Read the model definition and answer for the solid it produces. Units are mm, in the model's axes. Face numbers are marked on the shaded views. A direction names the side the tool comes from. Give positions to 0.01 mm unless a question says otherwise; leave off trailing zeros. Write each loop counter-clockwise with the first axis right and the second up, starting at its lowest first coordinate (ties: lowest second). Pieces come first, ordered by that corner, then holes. Notation, with made-up numbers: M -19,2 L 15,2 A19 ccw 15,12 Z; hole C 68,33.25 d5. An arc over 180 degrees is marked long. Answer as CSV lines item,"result". Start each with the question number.
Autodesk Inventor part; units mm, degrees
ref_plane "YZ Plane" through (0, 0, 0) normal (1, 0, 0) x (0, 1, 0)
ref_plane "XZ Plane" through (0, 0, 0) normal (0, 1, 0) x (-1, 0, 0)
ref_plane "XY Plane" through (0, 0, 0) normal (0, 0, 1) x (1, 0, 0)
sketch "Sketch1" plane through (0, 0, 0) normal (0, 0, 1) x (1, 0, 0)
  line L0 (0, 0) -> (0, 38.4841) construction
  line L1 (2.8, 25) -> (3.8, 24)
  line L2 (3.8, 24) -> (3.8, 0)
  line L3 (2.8, 25) -> (1.4, 25)
  line L4 (1.4, 25) -> (1.4, 0)
  line L5 (1.4, 0) -> (3.8, 0)
  dimension "d1" = 1.4
  dimension "d8" = 1
  dimension "d20" = 3.8
revolve "Revolution1" add sketch "Sketch1" angle 360 about axis through (0, 0, 0) along (0, 1, 0)
chamfer "Chamfer1" distance 0.5 angle 45 2 edges at (-1.4, 25, 0) (-1.4, 0, 0)
sketch "Sketch6" plane through (0, 0, 0) normal (0, -1, 0) x (1, 0, 0)
  line L0 (0, 0) -> (0, -8) construction
  circle A0 centre (0, 8) radius 3
  circle A1 centre (0, -8) radius 3
  circle A2 centre (0, 0) radius 6
  line L1 (0, 0) -> (0, 8) construction
  circle A3 centre (0, 8) radius 1.35
  circle A4 centre (0, -8) radius 1.35
  circle A5 centre (0, 0) radius 1.9
  point P0 (1.9111, -5.6875)
  point P1 (1.9111, 5.6875)
  point P2 (-1.9111, 5.6875)
  point P3 (-1.9111, -5.6875)
  dimension "d24" = 6
  dimension "d26" = 8
  dimension "d27" = 12
  dimension "d28" = 2.7
extrude "Extrusion3" add sketch "Sketch6" against normal blind 8
fillet "Fillet1" radius 4 4 edges at (1.9111, 4, 5.6875) (-1.9111, 4, 5.6875) (1.9111, 4, -5.6875) (-1.9111, 4, -5.6875)
fillet "Fillet2" radius 0.5 4 edges at (0, 8, -11) (6, 8, 0) (-6, 8, 0) (0, 8, 11)
properties part number "caster-bng"
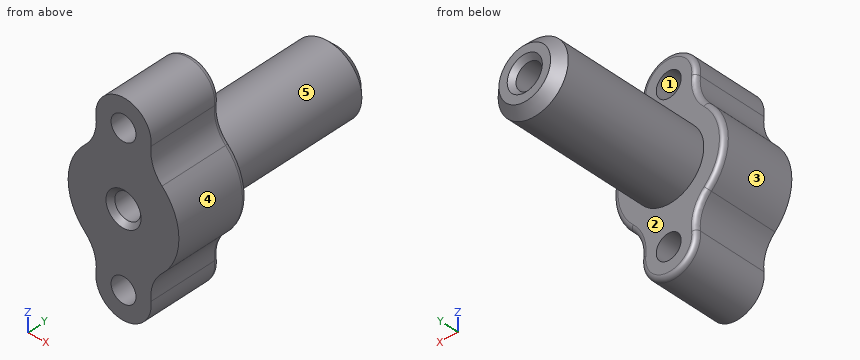
1. Find section D-D on z = 0. Determine the outline of the cut face in (x, y), then the cut area to 3 significant figures.
2. Find section A-A on z = -8. Determine the outline of the cut face in (x, y), then the cut area to 3 significant figures.
3. Find section B-B on x = 0. Determine the outline of the cut face in (y, z).
4. Find the intervals of material crossed by line 1 (Z direction, x = 0, y = 6.75); line 2 (X direction, y = 22.25, z = 0), in increasing order. Write a range as [from, to].
5. For the marked faces 4 and 5, determine the directions among +Z, -Z, +X, -X, +Y, -Y from which every point of the face is accessible in a straight line to the end or side of a thin tool.
6. Determine the mould class of the marked faces 1, 2 and 3 for opening direction Z: +Z half, -Z half, draft (parallel to the pull), parting line (faces both ways), or undercut.
7. Find section C-C on y = 19. Determine the outline of the cut face in (x, z), then the cut area to 3 significant figures.
8. Given pin 1 (1.5 mm diameter, centred on x = 2.5, y = 15, fed in from +Z); pin 2 (6 mm diameter, centred on x = -2.5, y = 12.5, fed in from +Z); pin 3 (1.6 mm diameter, centred on x = 0, z = 8, fed in from +Y); pin 4 (3.5 mm diameter, centred on x = 0, z = 0, fed in from +Y), each flat-ended and moving along its own axis, determine where each tip first touches the part or whether it passes through.
Computed:
1,outline,"M -6,0 L -1.9,0 L -1.4,0.5 L -1.4,24.5 L -1.9,25 L -2.8,25 L -3.8,24 L -3.8,8 L -5.5,8 A0.5 ccw -6,7.5 Z; M 1.4,0.5 L 1.9,0 L 6,0 L 6,7.5 A0.5 ccw 5.5,8 L 3.8,8 L 3.8,24 L 2.8,25 L 1.9,25 L 1.4,24.5 Z"
1,area,"154 mm^2"
2,outline,"M -3,0 L -1.35,0 L -1.35,8 L -2.5,8 A0.5 ccw -3,7.5 Z; M 1.35,0 L 3,0 L 3,7.5 A0.5 ccw 2.5,8 L 1.35,8 Z"
2,area,"26.3 mm^2"
3,outline,"M 0,-11 L 7.5,-11 A0.5 ccw 8,-10.5 L 8,-9.35 L 0,-9.35 Z; M 0,-6.65 L 8,-6.65 L 8,-3.8 L 24,-3.8 L 25,-2.8 L 25,-1.9 L 24.5,-1.4 L 0.5,-1.4 L 0,-1.9 Z; M 0,1.9 L 0.5,1.4 L 24.5,1.4 L 25,1.9 L 25,2.8 L 24,3.8 L 8,3.8 L 8,6.65 L 0,6.65 Z; M 0,9.35 L 8,9.35 L 8,10.5 A0.5 ccw 7.5,11 L 0,11 Z"
4,line 1,"z = [-11, -9.35], [-6.65, -1.4], [1.4, 6.65], [9.35, 11]"
4,line 2,"x = [-3.8, -1.4], [1.4, 3.8]"
5,face 4,"+X, +Y, -Y"
5,face 5,"+Y"
6,face 1,"undercut"
6,face 2,"draft"
6,face 3,"parting line"
7,outline,"C 0,0 d7.6; hole C 0,0 d2.8"
7,area,"39.2 mm^2"
8,pin 1,"stops at z = 3.37"
8,pin 2,"stops at z = 3.8"
8,pin 3,"passes through"
8,pin 4,"stops at y = 24.85"
